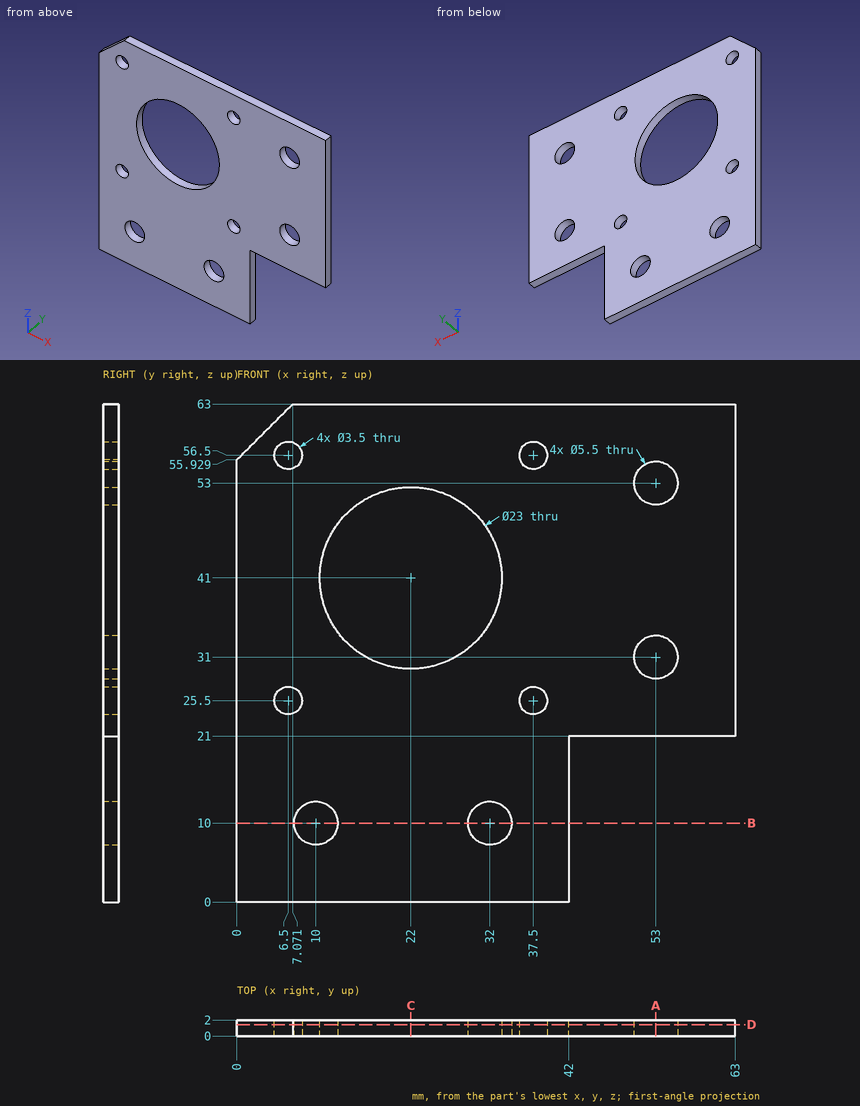
Answer from the drawing. Dimensions are ordinates in mm from the lowest x, y and z of the part. Coordinates: 2 decimals unless noted, no trailing zeros. Write each loop counter-clockwise with the first axis right and the second up, starting at its lowest first coordinate (ties: lowest second). Pieces come first, ordered by that corner, then holes. Notation, with made-up numbers: (35.5, -32.5) - (51.5, -32.5) arc R13 ccw to (51.5, -8.5) - close; hole circle Ø3 at (76.25, -6). An arc over 180 degrees is marked (long way). Return JSON: item names as keys, results as strings. Group by question number.
Q1. The part is cut by section C-C on x = 22. Write down the section's boundary in (y, z).
Q2. A flat-ended cylindrical pin translates along its axis: pin 1 Ø18.5 at (x, z) = (22, 41) entering from -Y. Find the tip coordinate at first contact, or state that the pin passes through.
Q3. Find the intervals of material crossed by line 1 along X through (y, z) = (1.2, 10); line 2 along X through (y, z) = (0.95, 41); line 3 along Z through (x, y) = (53, 0.85), in increasing order. Write a range as [from, to].
Q4. The part is cut by section D-D on y = 1.45. State how many separate pieces and enclosed holes the cut face has, and give its area (3 significant figures).
Q5. The part is cut by section A-A on x = 53. Write down the section's boundary in (y, z), and give its area (3 significant figures).
Q6. The part is cut by section B-B on z = 10. Write down the section's boundary in (x, y).
Evaluation:
{
 "1": {"outline": "(0, 0) - (2, 0) - (2, 29.5) - (0, 29.5) - close; (0, 52.5) - (2, 52.5) - (2, 63) - (0, 63) - close"},
 "2": {"pin 1": "passes through"},
 "3": {"line 1": "x = [0, 7.25], [12.75, 29.25], [34.75, 42]", "line 2": "x = [0, 10.5], [33.5, 63]", "line 3": "z = [21, 28.25], [33.75, 50.25], [55.75, 63]"},
 "4": {"separate pieces": "1", "enclosed holes": "9", "area": "2,950 mm2"},
 "5": {"outline": "(0, 21) - (2, 21) - (2, 28.25) - (0, 28.25) - close; (0, 33.75) - (2, 33.75) - (2, 50.25) - (0, 50.25) - close; (0, 55.75) - (2, 55.75) - (2, 63) - (0, 63) - close", "area": "62.0 mm2"},
 "6": {"outline": "(0, 0) - (7.25, 0) - (7.25, 2) - (0, 2) - close; (12.75, 0) - (29.25, 0) - (29.25, 2) - (12.75, 2) - close; (34.75, 0) - (42, 0) - (42, 2) - (34.75, 2) - close"}
}
